Input: part model. Units: mm. Frame: model coordinates. Face numbers are marked on the shaded views. A direction names the side the tool comes from. Coordinates: 2 decimals unless noted, no trailing zeros. Write each loop counter-clockwise with the first axis right and the second up, starting at its lowest first coordinate (ties: lowest second). Pieces come first, ordered by that corner, then holes.
1) Section query B-B (x = -11.75). Output: boundary loops of the cut face in (y, z).
2) Set-up query: the marked faces 4, 5, 6, 7 and 8. Return all of +Z, -Z, +X, -X, +Y, -Y with unobstructed straight access to the full face (end or side cutting, diameter ignored); none if empty.
3) Draft query along Y for the marked faces 1, 2 and 3. Return one class per face: pulls with the +Y half, pulls with the -Y half, needs draft (parallel to the pull), parting line crosses it, or undercut.
4) Section query A-A (x = -15). Output: boundary loops of the cut face in (y, z).
5) Line query: L1, parallel to Y at x = -15, z = 0; L2, parallel to Y at x = -12.25, z = 0; L3, parallel to X at y = 3.25, z = -6.5. Output: solid intervals per line, ascending.
6) Pin query (flat end, axial travel): pin 1 Ø0.6 at (x, z) = (-21.5, 5.5) entering from -Y; pin 2 Ø1.5 at (x, y) = (-13, -2.5) entering from +Z; pin 3 Ø2 at (y, z) = (-0.5, -6) entering from -X; pin 4 Ø2 at (y, z) = (0, -2.5) entering from -X. Return the tip coordinate at first contact, or that it passes through.
from build123d import *

# Parameters (mm, degrees)
CUT_EXTRUDE_START        = -10
CUT_EXTRUDE_1_DEPTH      = 10
CUT_EXTRUDE_2_DEPTH      = 29.603774074
CUT_EXTRUDE_2_DEPTH_BACK = 29.603774074
SKETCH_3_W               = 1.4
SKETCH_3_H               = 5.5


with BuildPart() as part:
    # Эскиз1 → Повернуть1 (revolve)
    with BuildSketch(Plane(origin=(0, 0, 0), x_dir=(1, 0, 0), z_dir=(0, 1, 0)), mode=Mode.PRIVATE) as revolve_1_sk:
        with BuildLine():
            Line((-8.642542558, -6.5), (-8.642542558, -5))
            Line((-8.642542558, -5), (-21.642542558, -5))
            Line((-21.642542558, -5), (-21.642542558, -8.1))
            Line((-21.642542558, -8.1), (-20.920854721, -9.35))
            Line((-20.920854721, -9.35), (-17.642542558, -9.35))
            Line((-17.642542558, -9.35), (-17.642542558, -7.94))
            ThreePointArc((-17.642542558, -7.94), (-17.349649339, -7.232893219), (-16.642542558, -6.94))
            Line((-16.642542558, -6.94), (-14.142542558, -6.94))
            ThreePointArc((-14.142542558, -6.94), (-13.788989167, -7.086446609), (-13.642542558, -7.44))
            Line((-13.642542558, -7.44), (-13.082542558, -8))
            Line((-13.082542558, -8), (-10.142542558, -8))
            Line((-10.142542558, -8), (-8.642542558, -6.5))
        make_face()
    revolve(revolve_1_sk.sketch.rotate(Axis((24.823529412, 0, 0), (-1, 0, 0)), 180), axis=Axis((24.823529412, 0, 0), (-1, 0, 0)))

    # Эскиз2 → Вырез-Вытянуть1 (cut)
    with BuildSketch(Plane.ZY.offset(21.642542558).offset(CUT_EXTRUDE_START)):
        with BuildLine():
            Line((-8.097337525, 0.207665597), (-8.097337525, 4.675))
            ThreePointArc((-8.097337525, 4.675), (-9.35, 0), (-8.097337525, -4.675))
            Line((-8.097337525, -4.675), (-8.097337525, -0.207665597))
            ThreePointArc((-8.097337525, -0.207665597), (-8.1, 0), (-8.097337525, 0.207665597))
        make_face()
        with BuildLine():
            Line((-3.868825081, 7.116332798), (0, 9.35))
            ThreePointArc((0, 9.35), (-4.675, 8.097337525), (-8.097337525, 4.675))
            Line((-8.097337525, 4.675), (-4.228512445, 6.908667202))
            ThreePointArc((-4.228512445, 6.908667202), (-4.05, 7.014805771), (-3.868825081, 7.116332798))
        make_face()
        with BuildLine():
            ThreePointArc((8.097337525, 4.675), (4.675, 8.097337525), (0, 9.35))
            Line((0, 9.35), (3.868825081, 7.116332798))
            ThreePointArc((3.868825081, 7.116332798), (4.05, 7.014805771), (4.228512445, 6.908667202))
            Line((4.228512445, 6.908667202), (8.097337525, 4.675))
        make_face()
        with BuildLine():
            ThreePointArc((9.35, 0), (9.031406476, 2.419958072), (8.097337525, 4.675))
            Line((8.097337525, 4.675), (8.097337525, 0.207665597))
            ThreePointArc((8.097337525, 0.207665597), (8.099334354, 0.103841332), (8.1, 0))
            ThreePointArc((8.1, 0), (8.099334354, -0.103841332), (8.097337525, -0.207665597))
            Line((8.097337525, -0.207665597), (8.097337525, -4.675))
            ThreePointArc((8.097337525, -4.675), (9.031406476, -2.419958072), (9.35, 0))
        make_face()
        with BuildLine():
            ThreePointArc((0, -9.35), (4.675, -8.097337525), (8.097337525, -4.675))
            Line((8.097337525, -4.675), (4.228512445, -6.908667202))
            ThreePointArc((4.228512445, -6.908667202), (4.05, -7.014805771), (3.868825081, -7.116332798))
            Line((3.868825081, -7.116332798), (0, -9.35))
        make_face()
        with BuildLine():
            Line((-4.228512445, -6.908667202), (-8.097337525, -4.675))
            ThreePointArc((-8.097337525, -4.675), (-4.675, -8.097337525), (0, -9.35))
            Line((0, -9.35), (-3.868825081, -7.116332798))
            ThreePointArc((-3.868825081, -7.116332798), (-4.05, -7.014805771), (-4.228512445, -6.908667202))
        make_face()
    extrude(amount=CUT_EXTRUDE_1_DEPTH, mode=Mode.SUBTRACT)

    # Эскиз3 → Вырез-Вытянуть2 (cut, two sides: drawn at the far end of the back side and taken through both)
    with BuildSketch(Plane(origin=(0, 0, -8.097337525), x_dir=(-1, 0, 0), z_dir=(0, 0, -1)).offset(-CUT_EXTRUDE_2_DEPTH_BACK)):
        with Locations((21.642542558, 0)):
            Rectangle(SKETCH_3_W, SKETCH_3_H)
    extrude(amount=CUT_EXTRUDE_2_DEPTH + CUT_EXTRUDE_2_DEPTH_BACK, mode=Mode.SUBTRACT)


solid = part.part
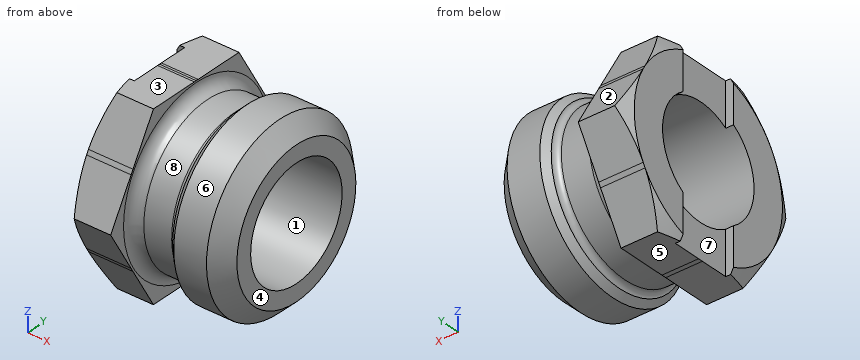
Answer:
1. outline: circle Ø16 at (0, 0); hole circle Ø10 at (0, 0)
2. face 4: +Z, -Z, +X, +Y, -Y
2. face 5: -Z, +X, -X, +Y, -Y
2. face 6: +X
2. face 7: +Z, -Z, -X
2. face 8: none
3. face 1: undercut
3. face 2: pulls with the +Y half
3. face 3: needs draft
4. outline: circle Ø13.88 at (0, 0); hole circle Ø10 at (0, 0)
5. L1: y = -6.94 to -5, 5 to 6.94
5. L2: y = -8 to -5, 5 to 8
5. L3: x = -21.64 to -17.38, -13.67 to -9.41
6. pin 1: stops at y = -6.35
6. pin 2: stops at z = 7.81
6. pin 3: stops at x = -20.94
6. pin 4: passes through
